Autodesk Inventor part; units mm, degrees
ref_plane "YZ Plane" through (0, 0, 0) normal (1, 0, 0) x (0, 1, 0)
ref_plane "XZ Plane" through (0, 0, 0) normal (0, 1, 0) x (-1, 0, 0)
ref_plane "XY Plane" through (0, 0, 0) normal (0, 0, 1) x (1, 0, 0)
sketch "Sketch1" plane through (0, 0, 0) normal (0, 1, 0) x (-1, 0, 0)
  circle A0 centre (0, 0) radius 9.5
  line L0 (3, 15) -> (-3, 15)
  line L1 (-3, -15) -> (3, -15)
  line L2 (-15, 3) -> (-15, -3)
  line L3 (15, -3) -> (15, 3)
  line L4 (3, -15) -> (3, -9.0139)
  line L5 (3, 9.0139) -> (3, 15)
  line L6 (15, 3) -> (9.0139, 3)
  line L7 (-9.0139, 3) -> (-15, 3)
  line L8 (-3, 15) -> (-3, 9.0139)
  line L9 (-3, -9.0139) -> (-3, -15)
  line L10 (-15, -3) -> (-9.0139, -3)
  line L11 (9.0139, -3) -> (15, -3)
  circle A1 centre (0, 0) radius 4
  point P0 (15, 0)
  point P1 (0, -15)
  point P2 (0, 15)
  point P3 (-15, 0)
  point P4 (9.5, 0)
  dimension "d0" = 19
  dimension "d2" = 6
  dimension "d7" = 5.5
  dimension "d10" = 8
extrude "Extrusion1" add sketch "Sketch1" along normal blind 6
fillet "Fillet1" radius 2 8 edges at (3, 3, 15) (-3, 3, 15) (-15, 3, 3) (-15, 3, -3) (-3, 3, -15) (3, 3, -15) (15, 3, -3) (15, 3, 3)
sketch "Sketch2" plane through (0, 6, 0) normal (0, 1, 0) x (1, 0, 0)
  line L0 (-6.5, 3.7528) -> (0, 7.5056)
  line L1 (0, 7.5056) -> (6.5, 3.7528)
  line L2 (6.5, 3.7528) -> (6.5, -3.7528)
  line L3 (6.5, -3.7528) -> (0, -7.5056)
  line L4 (0, -7.5056) -> (-6.5, -3.7528)
  line L5 (-6.5, -3.7528) -> (-6.5, 3.7528)
  line L6 (-15, 1) -> (-15, -1)
  point P0 (0, 0)
  point P1 (0, 0)
  dimension "d6" = 13
extrude "Extrusion2" cut sketch "Sketch2" against normal blind 5
properties part number "Wing_Nut"
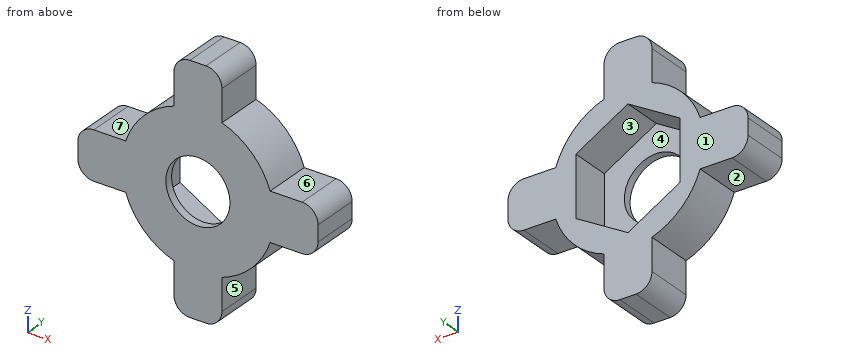
Input: part model. Units: mm. Frame: model coordinates. Face numbers are marked on the shaded views. A direction names the side the tool comes from. Give positions to 0.01 mm unless a question says otherwise; leave off trailing zeros. Order: outer loops, then holes, each group sorted by start corner. A loop starts at its lowest first (then second) coordinate and runs counter-clockwise, first axis right, second up.
Q1. Set-up query: the marked faces 5, 6 and 7. Return all of +Z, -Z, +X, -X, +Y, -Y with unobstructed straight access to the full face (end or side cutting, diameter ignored); none if empty.
Checked values:
face 5: -Z, +X, +Y, -Y
face 6: +Z, +X, +Y, -Y
face 7: +Z, -X, +Y, -Y
Q2. Ray query, probe 1 along Z at (x, y) = (0, 0.6); probe 2 along Y at (x, z) = (-3, 4.5). Return the intervals inside material, ascending.
Checked values:
probe 1: z = -15 to -4, 4 to 15
probe 2: y = 0 to 1
Q3. Draft query along Z for the marked faces 1, 2, 3 and 4. Return one class per face: +Z half, -Z half, draft (parallel to the pull), parting line (faces both ways), or undercut.
Checked values:
face 1: draft
face 2: -Z half
face 3: undercut
face 4: undercut
Q4. Section A-A on z = 0. Output: boundary loops of the cut face in (x, y), and give its area (3 significant figures).
Checked values:
outline: (-15, 0) - (-4, 0) - (-4, 1) - (-6.5, 1) - (-6.5, 6) - (-15, 6) - close; (4, 0) - (15, 0) - (15, 6) - (6.5, 6) - (6.5, 1) - (4, 1) - close
area: 107 mm2
Q5. Section D-D on x = 5.5. Output: boundary loops of the cut face in (y, z), and give its area (4 significant figures).
Checked values:
outline: (0, -7.75) - (6, -7.75) - (6, -4.33) - (1, -4.33) - (1, 4.33) - (6, 4.33) - (6, 7.75) - (0, 7.75) - close
area: 49.65 mm2
Q6. Contact query for flat-ended pins moving along their axis: pin 1 Ø2 at (y, z) = (3.5, -7.5) entering from +X; pin 2 Ø2 at (x, y) = (3, 1.5) entering from -Z; pin 3 Ø2 at (y, z) = (3, 11.5) entering from -X. Output: stop coordinate, or through.
Checked values:
pin 1: stops at x = 6.93
pin 2: stops at z = -14.73
pin 3: stops at x = -3
Q7. Section B-B on x = -0.5. Output: boundary loops of the cut face in (y, z).
Checked values:
outline: (0, -15) - (6, -15) - (6, -7.22) - (1, -7.22) - (1, -3.97) - (0, -3.97) - close; (0, 3.97) - (1, 3.97) - (1, 7.22) - (6, 7.22) - (6, 15) - (0, 15) - close
